```python
from build123d import *

# Parameters (mm, degrees)
SKETCH1_W            = 54.5
SKETCH1_H            = 40.5
BOSS_EXTRUDE1_DEPTH  = 2.5
M5_CLEARANCE_HOLE1_D = 5.5
FILLET1_R            = 5
BOSS_EXTRUDE2_DEPTH  = 2.5
MIRROR2_COPY_1_DEPTH = 2.5


with BuildPart() as part:
    # Sketch1 → Boss-Extrude1 (new body)
    with BuildSketch(Plane(origin=(0, 0, 0), x_dir=(1, 0, 0), z_dir=(0, 1, 0))):
        Rectangle(SKETCH1_W, SKETCH1_H)
    extrude(amount=BOSS_EXTRUDE1_DEPTH)

    # M5 Clearance Hole1 (through all)
    with Locations(Plane(origin=(0, 2.5, 0), x_dir=(1, 0, 0), z_dir=(0, 1, 0))):
        with Locations((17.5, -12), (-17.5, 12), (-17.5, -12), (17.5, 12)):
            Hole(M5_CLEARANCE_HOLE1_D / 2)

    # Fillet1
    fillet1_edges = [part.edges().sort_by_distance(p)[0] for p in [
        (-27.25, 1.25, -20.25),
        (27.25, 1.25, -20.25),
        (27.25, 1.25, 20.25),
        (-27.25, 1.25, 20.25),
    ]]
    fillet(fillet1_edges, radius=FILLET1_R)

    # Sketch2 → Boss-Extrude2 (add)
    with BuildSketch(Plane(origin=(0, 0, 0), x_dir=(1, 0, 0), z_dir=(0, 1, 0))):
        with BuildLine():
            Line((-25.25, 11), (-25.25, 15.25))
            ThreePointArc((-25.25, 15.25), (-26.25, 16.25), (-27.25, 15.25))
            Line((-27.25, 15.25), (-27.25, 11))
            ThreePointArc((-27.25, 11), (-26.25, 10), (-25.25, 11))
        make_face()
        with BuildLine():
            Line((-22.25, 18.25), (-18, 18.25))
            ThreePointArc((-18, 18.25), (-17, 19.25), (-18, 20.25))
            Line((-18, 20.25), (-22.25, 20.25))
            ThreePointArc((-22.25, 20.25), (-23.25, 19.25), (-22.25, 18.25))
        make_face()
    boss_extrude2 = extrude(amount=-BOSS_EXTRUDE2_DEPTH)

    # Mirror1: Boss-Extrude2 across plane
    add(boss_extrude2.mirror(Plane.XY))

    # Mirror2: Boss-Extrude2 across plane
    add(boss_extrude2.mirror(Plane(origin=(0, 0, 0), x_dir=(0, 0, 1), z_dir=(1, 0, 0))))

    # Mirror2 copy 1 sketch → Mirror2 copy 1 (add)
    with BuildSketch(Plane(origin=(0, 0, 0), x_dir=(-1, 0, 0), z_dir=(0, 1, 0))):
        with BuildLine():
            Line((-25.25, 11), (-25.25, 15.25))
            ThreePointArc((-25.25, 15.25), (-26.25, 16.25), (-27.25, 15.25))
            Line((-27.25, 15.25), (-27.25, 11))
            ThreePointArc((-27.25, 11), (-26.25, 10), (-25.25, 11))
        make_face()
        with BuildLine():
            Line((-22.25, 18.25), (-18, 18.25))
            ThreePointArc((-18, 18.25), (-17, 19.25), (-18, 20.25))
            Line((-18, 20.25), (-22.25, 20.25))
            ThreePointArc((-22.25, 20.25), (-23.25, 19.25), (-22.25, 18.25))
        make_face()
    extrude(amount=-MIRROR2_COPY_1_DEPTH)


solid = part.part
```
Check sheet for the modelled part. Datum: model origin and axes. Units: mm. A direction names the side the tool comes from. Coordinates: 2 decimals unless noted, no trailing zeros. Order: outer loops, then holes, each group sorted by start corner. A loop starts at its lowest first (then second) coordinate and runs counter-clockwise, first axis right, second up. Notation, with made-up numbers: (-15.75, -37.5) -> (28.25, -37.5) arc R30 ccw to (28.25, -9.5) -> close; hole circle Ø1 at (54.25, 71). An arc over 180 degrees is marked (long way). Write each question's results on one line, items separated by ' | '. Start each with the question number.
1) Material ranges on line 1 along Z through (x, y) = (17.5, 0.65); line 2 along X through (y, z) = (1.4, 12); line 3 along X through (y, z) = (1.7, -13.5), recorded low to high.
2) Set-up check for faces 4 (the face through (-25.25, -1, -13)), 5 (the face through (-20, -1, 18.25)), 6 (the face through (-23.25, -1.23, -19.27)), 7 (the face through (-26.3, -1.2, 10)): record each of +Z, -Z, +X, -X, +Y, -Y from which the full face is reachable in a straight line by a thin tool's end or side.
3) Section check A-A (y = -1.25). Count the separate pieces of the cut face and the enclosed holes in it, and give its area (3 significant figures).
4) Section check D-D (x = -21.5). Enter the section's corners in (y, z), and give its area (3 significant figures).
5) Section check C-C (z = 19.25). Enter the section's corners in (x, y).
6) Draft check along X on faces 1 (the face through (-20, -2.5, -19)), 2 (the face through (26.3, -1.2, -10)), 3 (the face through (-27.25, 1, 0)). Enter one of: pulls with the +X half, pulls with the -X half, needs draft (parallel to the pull), parting line crosses it, or undercut.
7) Depth check by flat-ended pin: pin 1 (6.5 mm diameter, centred on x = -17.5, z = 12, fed in from -Y). Enter the tip coordinate at first touch or a pass-through.
8) Section check B-B (x = 26.25). Enter the section's corners in (y, z).
Checked values:
1) line 1: -20.25 to -14.75, -9.25 to 9.25, 14.75 to 20.25 | line 2: -27.25 to -20.25, -14.75 to 14.75, 20.25 to 27.25 | line 3: -27.25 to -19.8, -15.2 to 15.2, 19.8 to 27.25
2) face 4: +Z, -Z, -Y | face 5: +X, -X, -Y | face 6: -X, -Y | face 7: -Y
3) separate pieces: 8 | enclosed holes: 0 | area: 93.1 mm²
4) outline: (-2.5, -20.25) -> (2.5, -20.25) -> (2.5, 20.25) -> (-2.5, 20.25) -> (-2.5, 18.25) -> (0, 18.25) -> (0, -18.25) -> (-2.5, -18.25) -> close | area: 111 mm²
5) outline: (-25.25, 0) -> (-23.25, 0) -> (-23.25, -2.5) -> (-17, -2.5) -> (-17, 0) -> (17, 0) -> (17, -2.5) -> (23.25, -2.5) -> (23.25, 0) -> (25.25, 0) -> (25.25, 2.5) -> (-25.25, 2.5) -> close
6) face 1: needs draft | face 2: undercut | face 3: pulls with the -X half
7) pin 1: y = 0
8) outline: (-2.5, -16.25) -> (0, -16.25) -> (0, -18.25) -> (2.5, -18.25) -> (2.5, 18.25) -> (0, 18.25) -> (0, 16.25) -> (-2.5, 16.25) -> (-2.5, 10) -> (0, 10) -> (0, -10) -> (-2.5, -10) -> close
